Input: dimensioned drawing with shaded views. Units: mm. Origin: part minimum x, y, z. A direction names the side the tool comes from. Round coordinates to 2 decimals unless told otherwise and drop trailing zeros. Order: outer loops, then holes, each group sorted by start corner. A loop starts at its lowest first (then second) coordinate and runs counter-clockwise, first axis right, second up. Notation, with made-up numbers: (77.25, 10) - (129.25, 10) arc R31 cw to (129.25, 47) - close; hole circle Ø2 at (51, 70). An arc over 180 degrees is marked (long way). Put each result on its own line as item: value. Start each with the question number.
(1) Section B-B (x = 35). Output: boundary loops of the cut face in (y, z), and give its area (3 significant figures).
(2) Section D-D (x = 16). Output: boundary loops of the cut face in (y, z).
(3) Access query for the marked faces 1 and 2. Directions: +Z, -Z, +X, -X, +Y, -Y. A direction counts if a zero-diameter tool reaches every point of the face in a straight line with its end or side. Return the directions, or none.
(4) Section C-C (z = 9). Output: boundary loops of the cut face in (x, y), and give its area (3 significant figures).
(5) Material intervals for L1, parallel to X at y = 6, z = 9.35; L2, parallel to X at y = 7.5, z = 9.25; L3, parallel to Y at x = 35, z = 9.6, sorted ascending. Write a range as [from, to].
(6) Pin query (flat end, axial travel): P1, Ø6, axis at x = 24.5, z = 3, coming from the -Y side; P2, Ø5.5, axis at x = 5, y = 6, coming from the -Z side; P3, Ø3, axis at y = 8.5, z = 6, coming from the +X side. Return the tip coordinate at first contact, or that it passes through.
(7) Section A-A (y = 6). Output: boundary loops of the cut face in (x, z), and give its area (3 significant figures).
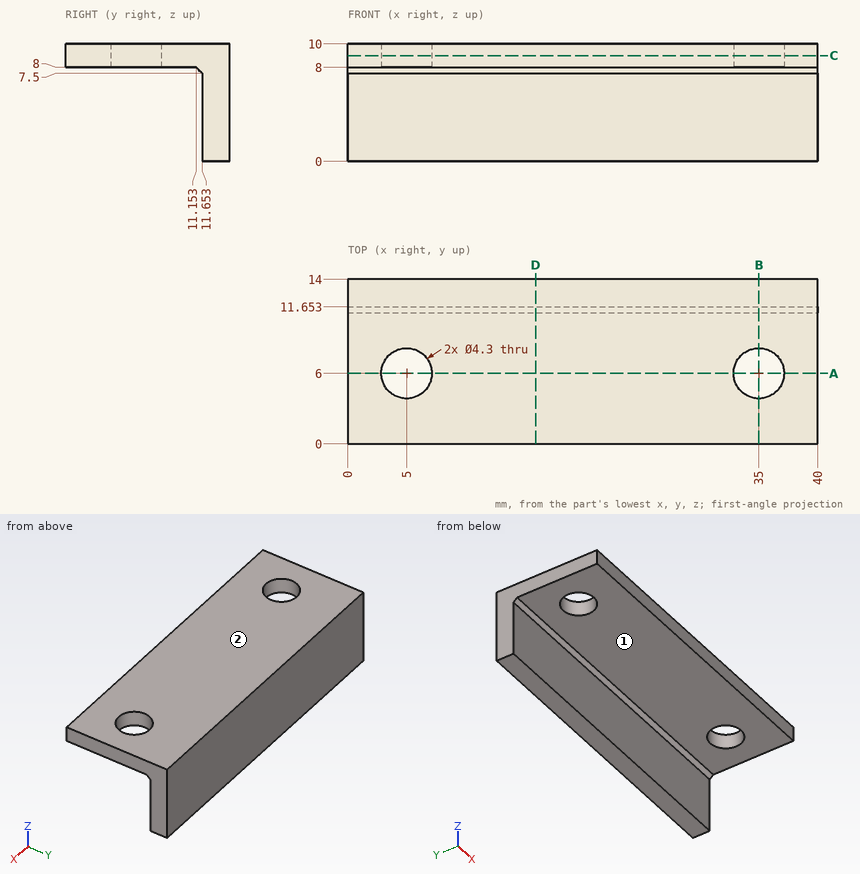
Checks:
1. outline: (0, 8) - (3.85, 8) - (3.85, 10) - (0, 10) - close; (8.15, 8) - (11.15, 8) - (11.65, 7.5) - (11.65, 0) - (14, 0) - (14, 10) - (8.15, 10) - close
1. area: 38.3 mm²
2. outline: (0, 8) - (11.15, 8) - (11.65, 7.5) - (11.65, 0) - (14, 0) - (14, 10) - (0, 10) - close
3. face 1: -Z, +X, -X, -Y
3. face 2: +Z, +X, -X, +Y, -Y
4. outline: (0, 0) - (40, 0) - (40, 14) - (0, 14) - close; hole circle Ø4.3 at (5, 6); hole circle Ø4.3 at (35, 6)
4. area: 531 mm²
5. L1: x = [0, 2.85], [7.15, 32.85], [37.15, 40]
5. L2: x = [0, 3.46], [6.54, 33.46], [36.54, 40]
5. L3: y = [0, 3.85], [8.15, 14]
6. P1: stops at y = 11.65
6. P2: stops at z = 8
6. P3: passes through
7. outline: (0, 8) - (2.85, 8) - (2.85, 10) - (0, 10) - close; (7.15, 8) - (32.85, 8) - (32.85, 10) - (7.15, 10) - close; (37.15, 8) - (40, 8) - (40, 10) - (37.15, 10) - close
7. area: 62.8 mm²
